CAD build for the part. Positions are in the model's coordinates, mm. Give positions to 0.01 mm unless a question says otherwise; leave off trailing zeros. Write each loop counter-clockwise with the first axis right and the second up, starting at its lowest first coordinate (ties: lowest second). Pieces come first, ordered by that corner, then holes. Notation, with made-up numbers: (-6.5, -36) -> (21.5, -36) arc R31 ccw to (21.5, -5) -> close; hole circle Ø7 at (46, -15). An arc over 180 degrees is marked (long way). Answer as a JSON object with one key per item and string values.
```python
from build123d import *

# Parameters (mm, degrees)
CIRCLE004_R      = 3.55
EXTRUDE004_DEPTH = 10
CIRCLE002_R      = 1.753689
EXTRUDE003_DEPTH = 10
CIRCLE001_R      = 1.746402
EXTRUDE002_DEPTH = 10
CIRCLE003_R      = 1.746988
EXTRUDE_DEPTH    = 10
CIRCLE_R         = 1.749447
EXTRUDE001_DEPTH = 10
BOX_W            = 45.2
BOX_H            = 20
BOX_DEPTH        = 2


with BuildPart() as extrude004:
    # Circle004 → Extrude004 (new body)
    with BuildSketch(Plane(origin=(30.45, 10, 2), x_dir=(-1, 0, 0), z_dir=(0, 0, 1))):
        Circle(CIRCLE004_R)
    extrude(amount=EXTRUDE004_DEPTH)


with BuildPart() as extrude004_1:
    # Extrude004 placement: moved
    add(extrude004.part.moved(Location((0, 0, -4))))


with BuildPart() as extrude003:
    # Circle002 → Extrude003 (new body)
    with BuildSketch(Plane(origin=(42.2, 17.004963, 2), x_dir=(-1, 0, 0), z_dir=(0, 0, 1))):
        Circle(CIRCLE002_R)
    extrude(amount=EXTRUDE003_DEPTH)


with BuildPart() as extrude003_1:
    # Extrude003 placement: moved
    add(extrude003.part.moved(Location((0, 0, -5))))


with BuildPart() as extrude002:
    # Circle001 → Extrude002 (new body)
    with BuildSketch(Plane(origin=(42.199112, 2.997812, 2), x_dir=(-1, 0, 0), z_dir=(0, 0, 1))):
        Circle(CIRCLE001_R)
    extrude(amount=EXTRUDE002_DEPTH)


with BuildPart() as extrude002_1:
    # Extrude002 placement: moved
    add(extrude002.part.moved(Location((0, 0, -5))))


with BuildPart() as extrude_body:
    # Circle003 → Extrude (new body)
    with BuildSketch(Plane(origin=(3, 17.004963, 2), x_dir=(-1, 0, 0), z_dir=(0, 0, 1))):
        Circle(CIRCLE003_R)
    extrude(amount=EXTRUDE_DEPTH)


with BuildPart() as extrude_body_1:
    # Extrude placement: moved
    add(extrude_body.part.moved(Location((0, 0, -5))))


with BuildPart() as extrude001:
    # Circle → Extrude001 (new body)
    with BuildSketch(Plane(origin=(3, 2.998732, 2), x_dir=(-1, 0, 0), z_dir=(0, 0, 1))):
        Circle(CIRCLE_R)
    extrude(amount=EXTRUDE001_DEPTH)


with BuildPart() as extrude001_1:
    # Extrude001 placement: moved
    add(extrude001.part.moved(Location((0, 0, -5))))


with BuildPart() as base_con_agujeros:
    # Box → Box (new body)
    with BuildSketch(Plane.XY):
        with Locations((22.6, 10)):
            Rectangle(BOX_W, BOX_H)
    extrude(amount=BOX_DEPTH)

    # Cut: cut Extrude001
    add(extrude001_1.part, mode=Mode.SUBTRACT)

    # Cut001: cut Extrude body
    add(extrude_body_1.part, mode=Mode.SUBTRACT)

    # Cut002: cut Extrude002
    add(extrude002_1.part, mode=Mode.SUBTRACT)

    # Cut003: cut Extrude003
    add(extrude003_1.part, mode=Mode.SUBTRACT)

    # Cut004: cut Extrude004
    add(extrude004_1.part, mode=Mode.SUBTRACT)


solid = base_con_agujeros.part
```
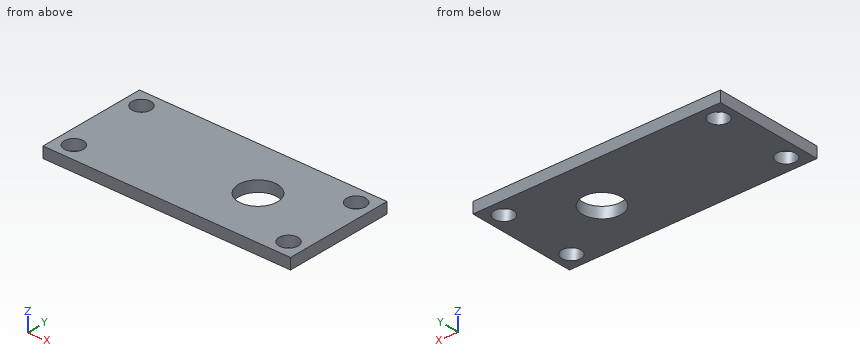
1) Slice it at D-D (y = 16.25). List the corners of the cut face in (x, z), then the cut area to 3 significant figures.
Model answer:
{"outline": "(0, 0) -> (1.42, 0) -> (1.42, 2) -> (0, 2) -> close; (4.58, 0) -> (40.62, 0) -> (40.62, 2) -> (4.58, 2) -> close; (43.78, 0) -> (45.2, 0) -> (45.2, 2) -> (43.78, 2) -> close", "area": "77.8 mm2"}
2) Slice it at C-C (x = 3). List the corners of the cut face in (y, z).
Model answer:
{"outline": "(0, 0) -> (1.25, 0) -> (1.25, 2) -> (0, 2) -> close; (4.75, 0) -> (15.26, 0) -> (15.26, 2) -> (4.75, 2) -> close; (18.75, 0) -> (20, 0) -> (20, 2) -> (18.75, 2) -> close"}
3) Wall check: probe 1 along Y at (x, z) = (3, 1.05); probe 2 along Y at (x, z) = (42.2, 0.55); probe 3 along X at (y, z) = (13, 0.3). Give the ranges that are in metal, low to high.
Model answer:
{"probe 1": "y = 0 to 1.25, 4.75 to 15.26, 18.75 to 20", "probe 2": "y = 0 to 1.25, 4.74 to 15.25, 18.76 to 20", "probe 3": "x = 0 to 28.55, 32.35 to 45.2"}
4) Slice it at A-A (x = 30.45). List the corners of the cut face in (y, z), then the cut area to 3 significant figures.
Model answer:
{"outline": "(0, 0) -> (6.45, 0) -> (6.45, 2) -> (0, 2) -> close; (13.55, 0) -> (20, 0) -> (20, 2) -> (13.55, 2) -> close", "area": "25.8 mm2"}
5) Slice it at B-B (y = 10). List the corners of the cut face in (x, z), then the cut area to 3 significant figures.
Model answer:
{"outline": "(0, 0) -> (26.9, 0) -> (26.9, 2) -> (0, 2) -> close; (34, 0) -> (45.2, 0) -> (45.2, 2) -> (34, 2) -> close", "area": "76.2 mm2"}
